The listing builds one solid part. Answer for the finished solid, in the listing's coordinates (mm). A direction names the side the tool comes from. Coordinates: 2 decimals unless noted, no trailing zeros. Write each loop counter-clockwise with the first axis right and the second up, starting at its lowest first coordinate (ties: lowest second). Pieces come first, ordered by that corner, then holes. Notation, with made-up numbers: M -1.75,2.25 L 49.25,2.25 A34 cw 49.25,41.25 Z; hole C -35,-8.5 d11. An arc over 180 degrees is marked long. Put each result on its own line as item: value. Start each with the question number.
```python
from build123d import *

# Parameters (mm, degrees)
ESBO_O1_W                = 30
ESBO_O1_H                = 10
RESSALTO_EXTRUS_O1_DEPTH = 5
ESBO_O2_W                = 5.2
ESBO_O2_H                = 5.2
CORTE_EXTRUS_O1_DEPTH    = 2.7
CHANFRO1_SIZE            = 0.7
FILETE1_R                = 2
FILETE2_R                = 2
FILETE3_R                = 2
FILETE4_R                = 2


with BuildPart() as part:
    # Esboço1 → Ressalto-extrusão1 (new body)
    with BuildSketch(Plane(origin=(0, 0, 0), x_dir=(1, 0, 0), z_dir=(0, 1, 0))):
        with Locations((15, 5)):
            Rectangle(ESBO_O1_W, ESBO_O1_H)
    extrude(amount=RESSALTO_EXTRUS_O1_DEPTH)

    # Esboço2 → Corte-extrusão1 (cut)
    with BuildSketch(Plane(origin=(0, 5, 0), x_dir=(1, 0, 0), z_dir=(0, 1, 0))):
        with Locations((6, 5)):
            Rectangle(ESBO_O2_W, ESBO_O2_H)
    extrude(amount=-CORTE_EXTRUS_O1_DEPTH, mode=Mode.SUBTRACT)

    # Chanfro1
    chanfro1_edges = [part.edges().sort_by_distance(p)[0] for p in [
        (8.6, 5, -5),
        (6, 5, -7.6),
        (3.4, 5, -5),
        (6, 5, -2.4),
    ]]
    chamfer(chanfro1_edges, length=CHANFRO1_SIZE)

    # Filete1
    filete1_edges = [part.edges().sort_by_distance(p)[0] for p in [
        (30, 2.5, 0),
    ]]
    fillet(filete1_edges, radius=FILETE1_R)

    # Filete2
    filete2_edges = [part.edges().sort_by_distance(p)[0] for p in [
        (30, 2.5, -10),
    ]]
    fillet(filete2_edges, radius=FILETE2_R)

    # Filete3
    filete3_edges = [part.edges().sort_by_distance(p)[0] for p in [
        (0, 2.5, 0),
    ]]
    fillet(filete3_edges, radius=FILETE3_R)

    # Filete4
    filete4_edges = [part.edges().sort_by_distance(p)[0] for p in [
        (0, 2.5, -10),
    ]]
    fillet(filete4_edges, radius=FILETE4_R)


solid = part.part
```
1) A cutting plane is placed at B-B on y = 3.2. Write down the section's boundary in (x, z), then the cut area to 3 significant figures.
2) A cutting plane is placed at C-C on x = 3. Write down the section's boundary in (y, z), then the cut area to 3 significant figures.
3) Determine the mould class of faces 3 (the face through (6, 2.3, -5)), 4 (the face through (15, 5, -5)), 5 (the face through (29.43, 2.54, -9.4)) for opening direction Z: +Z half, -Z half, draft (parallel to the pull), parting line (faces both ways), or undercut.
4) For faces 1 (the face through (15, 0, -5)), 2 (the face through (8.6, 3, -5)), determine the directions among +Z, -Z, +X, -X, +Y, -Y from which every point of the face is accessible in a straight line to the end or side of a thin tool.
5) A cutting plane is placed at D-D on z = -9. Write down the section's boundary in (x, y).
6) Given pin 1 Ø2.5 at (x, z) = (6, -5) entering from +Y, flat-ended and moving along its own axis, determine where the tip first touches the part or whether it passes through.
7) A cutting plane is placed at A-A on z = -4. Write down the section's boundary in (x, y).
8) Straight lines are drawn through the part: probe 1 along X at (y, z) = (4.55, -3.5); probe 2 along Y at (x, z) = (7, -5.5); probe 3 along Z at (x, y) = (7.25, 4.75). For each, find the intervals that lie inside material, in ascending order.
Answers follow:
1. outline: M 0,-8 A2 ccw 2,-10 L 28,-10 A2 ccw 30,-8 L 30,-2 A2 ccw 28,0 L 2,0 A2 ccw 0,-2 Z; hole M 3.4,-7.6 L 8.6,-7.6 L 8.6,-2.4 L 3.4,-2.4 Z
1. area: 270 mm²
2. outline: M 0,-10 L 5,-10 L 5,-8.3 L 4.7,-8 L 4.7,-2 L 5,-1.7 L 5,0 L 0,0 Z
2. area: 48.1 mm²
3. face 3: undercut
3. face 4: draft
3. face 5: -Z half
4. face 1: +Z, -Z, +X, -X, -Y
4. face 2: +Y
5. outline: M 0.27,0 L 29.73,0 L 29.73,5 L 0.27,5 Z
6. pin 1: stops at y = 2.3
7. outline: M 0,0 L 30,0 L 30,5 L 9.3,5 L 8.6,4.3 L 8.6,2.3 L 3.4,2.3 L 3.4,4.3 L 2.7,5 L 0,5 Z
8. probe 1: x = 0 to 3.15, 8.85 to 30
8. probe 2: y = 0 to 2.3
8. probe 3: z = -10 to -8.05, -1.95 to 0
